Can you work these out from the model? Positions are in its coordinate system, mm. A direction names the side the tool comes from. Round coordinates to 2 decimals unless told otherwise and drop trailing zeros. Loops run counter-clockwise (first coordinate to the right, second up) from the corner with the lowest first, then second, coordinate; pieces in that order, holes last. Notation, with made-up numbers: (-24.75, -8) -> (-0.75, -8) arc R28 ccw to (-0.75, 23) -> close; hole circle Ø1 at (84, 24). An arc over 180 degrees is marked (long way). Write item = value, one per line.
from build123d import *

# Parameters (mm, degrees)
MAIN_EXTRUDE_DEPTH          = 2.2875
WALLS_START                 = 2.2875
WALLS_DEPTH                 = 13
CORNER_SUPPORT_DEPTH        = 2
FILLET4_R                   = 2
SKETCH4_W                   = 8.5
SKETCH4_H                   = 5.5
WIRE_HOLE_DEPTH             = 40.380356778
SKETCH25_W                  = 6
SKETCH25_H                  = 1.35
FEMALE_SNAP_DEPTH           = 10.125
SKETCH30_W                  = 15.7875
SKETCH30_H                  = 0.9
SKETCH30_W_2                = 17.7875
SKETCH30_H_2                = 1.5
MAGNET_EXTRUDE_1_DEPTH      = 7.625
MAGNET_EXTRUDE_1_DEPTH_BACK = 8.2
SKETCH29_R                  = 7.7
MAGNET_HOLE_DEPTH           = 2.1
SKETCH31_R                  = 5.5
MAGNET_THRU_HOLE_DEPTH      = 58.632218908
SKETCH40_W                  = 15.2875
SKETCH40_H                  = 12.55
CUT_EXTRUDE2_DEPTH          = 6
SKETCH41_W                  = 13
SKETCH41_H                  = 2
BOSS_EXTRUDE1_DEPTH         = 9.4


with BuildPart() as part:
    # Sketch1 → Main Extrude (new body)
    with BuildSketch(Plane(origin=(0, 0, 0), x_dir=(0, 0, -1), z_dir=(1, 0, 0))):
        Polygon((-30.5, -9.35), (-27.325, -9.35), (-27.325, -21.25), (28.5, -21.25), (28.5, 21.25), (-27.325, 21.25), (-27.325, 3.2), (-30.5, 3.2), align=None)
        with BuildLine():
            Line((20.7, -3.65), (-2.8, -3.65))
            ThreePointArc((-2.8, -3.65), (-4.6, -1.85), (-2.8, -0.05))
            Line((-2.8, -0.05), (20.7, -0.05))
            ThreePointArc((20.7, -0.05), (22.5, -1.85), (20.7, -3.65))
        make_face(mode=Mode.SUBTRACT)
    extrude(amount=MAIN_EXTRUDE_DEPTH)

    # Sketch1_3 → Walls (add)
    with BuildSketch(Plane(origin=(0, 0, 0), x_dir=(0, 0, -1), z_dir=(1, 0, 0)).offset(WALLS_START)):
        Polygon((-25.325, 19.25), (28.5, 19.25), (28.5, 21.25), (-27.325, 21.25), (-27.325, 3.2), (-30.5, 3.2), (-30.5, 1.3), (-25.325, 1.3), align=None)
        with BuildLine():
            Line((28.5, -5.425), (28, -5.425))
            ThreePointArc((28, -5.425), (26.939339828, -5.864339828), (26.5, -6.925))
            Line((26.5, -6.925), (26.5, -19.25))
            Line((26.5, -19.25), (-25.325, -19.25))
            Line((-25.325, -19.25), (-25.325, -8.1))
            Line((-25.325, -8.1), (-28.5, -8.1))
            Line((-28.5, -8.1), (-28.5, -4.45))
            Line((-28.5, -4.45), (-30.5, -4.45))
            Line((-30.5, -4.45), (-30.5, -9.35))
            Line((-30.5, -9.35), (-27.325, -9.35))
            Line((-27.325, -9.35), (-27.325, -21.25))
            Line((-27.325, -21.25), (28.5, -21.25))
            Line((28.5, -21.25), (28.5, -5.425))
        make_face()
    extrude(amount=WALLS_DEPTH)

    # Sketch22 → Corner Support (add)
    with BuildSketch(Plane(origin=(0, 0, -28.5), x_dir=(-1, 0, 0), z_dir=(0, 0, -1))):
        Polygon((-4.2875, 19.25), (-2.2875, 18.25), (-2.2875, 19.25), align=None)
    extrude(amount=-CORNER_SUPPORT_DEPTH)

    # Fillet4
    fillet4_edges = [part.edges().sort_by_distance(p)[0] for p in [
        (2.2875, -1.575, 30.5),
    ]]
    fillet(fillet4_edges, radius=FILLET4_R)

    # Sketch4 → Wire Hole (cut, through all)
    with BuildSketch(Plane(origin=(2.2875, 0, 0), x_dir=(0, 0, -1), z_dir=(1, 0, 0))):
        with Locations((22.25, -16.5)):
            Rectangle(SKETCH4_W, SKETCH4_H)
    extrude(amount=-WIRE_HOLE_DEPTH, mode=Mode.SUBTRACT)

    # Sketch25 → Female Snap (cut, symmetric)
    with BuildSketch(Plane(origin=(0, 0, -0.5875), x_dir=(-1, 0, 0), z_dir=(0, 0, -1))):
        with Locations((-11.0375, -19.925)):
            Rectangle(SKETCH25_W, SKETCH25_H)
        Polygon((-15.2875, -19.25), (-15.2875, -19.91463679), (-14.0375, -19.25), align=None)
        with Locations((-11.0375, 19.925)):
            Rectangle(SKETCH25_W, SKETCH25_H)
        Polygon((-15.2875, 19.91463679), (-15.2875, 19.25), (-14.0375, 19.25), align=None)
    extrude(amount=FEMALE_SNAP_DEPTH, both=True, mode=Mode.SUBTRACT)

    # Sketch30 → Magnet Extrude 1 (add, two sides)
    with BuildSketch(Plane(origin=(15.2875, 0, 0), x_dir=(0, 0, -1), z_dir=(1, 0, 0))) as magnet_extrude_1_sk:
        Polygon((-27.325, -18.35), (-27.325, -21.25), (-9.5375, -21.25), (-9.5375, -19.91463679), (-9.5375, -19.25), (-25.325, -19.25), (-25.325, -18.35), align=None)
        with Locations((-17.43125, -18.8)):
            Rectangle(SKETCH30_W, SKETCH30_H)
        with Locations((19.60625, -22)):
            Rectangle(SKETCH30_W_2, SKETCH30_H_2)
        Polygon((10.7125, -19.91463679), (10.7125, -21.25), (28.5, -21.25), (28.5, -18.35), (26.5, -18.35), (26.5, -19.25), (10.7125, -19.25), align=None)
        with Locations((-18.43125, -22)):
            Rectangle(SKETCH30_W_2, SKETCH30_H_2)
        with Locations((18.60625, -18.8)):
            Rectangle(SKETCH30_W, SKETCH30_H)
    extrude(amount=MAGNET_EXTRUDE_1_DEPTH)
    extrude(magnet_extrude_1_sk.sketch, amount=-MAGNET_EXTRUDE_1_DEPTH_BACK)

    # Sketch29 → Magnet Hole (cut)
    with BuildSketch(Plane(origin=(0, -21.95, 0), x_dir=(1, 0, 0), z_dir=(0, 1, 0))):
        with Locations((15.2875, -17.625)):
            Circle(SKETCH29_R)
        with BuildLine():
            ThreePointArc((22.9125, -18.697089082), (20.338980677, -23.436414885), (15.2875, -25.325))
            Line((15.2875, -25.325), (22.9125, -25.325))
            Line((22.9125, -25.325), (22.9125, -18.697089082))
        make_face()
        with BuildLine():
            Line((22.9125, -9.925), (15.2875, -9.925))
            ThreePointArc((15.2875, -9.925), (20.338980677, -11.813585115), (22.9125, -16.552910918))
            Line((22.9125, -16.552910918), (22.9125, -9.925))
        make_face()
        with Locations((15.2875, 19.4)):
            Circle(SKETCH29_R)
        with BuildLine():
            ThreePointArc((22.9125, 18.327910918), (20.338980677, 13.588585115), (15.2875, 11.7))
            Line((15.2875, 11.7), (22.9125, 11.7))
            Line((22.9125, 11.7), (22.9125, 18.327910918))
        make_face()
        with BuildLine():
            Line((22.9125, 27.1), (15.2875, 27.1))
            ThreePointArc((15.2875, 27.1), (20.338980677, 25.211414885), (22.9125, 20.472089082))
            Line((22.9125, 20.472089082), (22.9125, 27.1))
        make_face()
        with BuildLine():
            ThreePointArc((22.9875, -17.625), (22.968727116, -17.087645368), (22.9125, -16.552910918))
            Line((22.9125, -16.552910918), (22.9125, -18.697089082))
            ThreePointArc((22.9125, -18.697089082), (22.968727116, -18.162354632), (22.9875, -17.625))
        make_face()
        with BuildLine():
            Line((22.9125, 20.472089082), (22.9125, 18.327910918))
            ThreePointArc((22.9125, 18.327910918), (22.968727116, 18.862645368), (22.9875, 19.4))
            ThreePointArc((22.9875, 19.4), (22.968727116, 19.937354632), (22.9125, 20.472089082))
        make_face()
    extrude(amount=MAGNET_HOLE_DEPTH, mode=Mode.SUBTRACT)

    # Sketch31 → Magnet Thru Hole (cut, through all)
    with BuildSketch(Plane.XZ.offset(21.95)):
        with Locations((15.2875, 17.625)):
            Circle(SKETCH31_R)
        with BuildLine():
            Line((22.9125, 23.125), (15.2875, 23.125))
            ThreePointArc((15.2875, 23.125), (19.176587297, 21.514087297), (20.7875, 17.625))
            ThreePointArc((20.7875, 17.625), (19.176587297, 13.735912703), (15.2875, 12.125))
            Line((15.2875, 12.125), (22.9125, 12.125))
            Line((22.9125, 12.125), (22.9125, 23.125))
        make_face()
        with Locations((15.2875, -19.4)):
            Circle(SKETCH31_R)
        with BuildLine():
            Line((22.9125, -13.9), (15.2875, -13.9))
            ThreePointArc((15.2875, -13.9), (19.176587297, -15.510912703), (20.7875, -19.4))
            ThreePointArc((20.7875, -19.4), (19.176587297, -23.289087297), (15.2875, -24.9))
            Line((15.2875, -24.9), (22.9125, -24.9))
            Line((22.9125, -24.9), (22.9125, -13.9))
        make_face()
    extrude(amount=MAGNET_THRU_HOLE_DEPTH, mode=Mode.SUBTRACT)

    # Sketch40 → Cut-Extrude2 (cut)
    with BuildSketch(Plane.XY.offset(27.325)):
        with Locations((7.64375, -3.075)):
            Rectangle(SKETCH40_W, SKETCH40_H)
    extrude(amount=CUT_EXTRUDE2_DEPTH, mode=Mode.SUBTRACT)

    # Sketch41 → Boss-Extrude1 (add)
    with BuildSketch(Plane.XZ.offset(-1.3)):
        with Locations((8.7875, 26.325)):
            Rectangle(SKETCH41_W, SKETCH41_H)
    extrude(amount=BOSS_EXTRUDE1_DEPTH)


solid = part.part
1. I'm going to push flat-ended pins straight in: pin 1 (0.7 mm diameter, centred on y = -19, z = 14, fed in from -X); pin 2 (20 mm diameter, centred on y = 3.5, z = -9.5, fed in from +X); pin 3 (3 mm diameter, centred on x = 3.5, z = 12.5, fed in from -Y); pin 4 (0.7 mm diameter, centred on y = 20, z = -4, fed in from +X). Where does each tip first touch, or does it pass through?
Entries:
pin_1 = 0
pin_2 = 2.29
pin_3 = -21.25
pin_4 = 15.29
2. Suppose I cut it at B-B, the plane z = -19.4. List the corners of the cut face in (x, y) for me.
Entries:
outline = (0, -21.25) -> (7.09, -21.25) -> (7.09, -22.75) -> (9.79, -22.75) -> (9.79, -21.95) -> (7.59, -21.95) -> (7.59, -19.85) -> (22.91, -19.85) -> (22.91, -18.35) -> (7.09, -18.35) -> (7.09, -19.25) -> (0, -19.25) -> close; (0, -13.75) -> (2.29, -13.75) -> (2.29, -3.65) -> (0, -3.65) -> close; (0, -0.05) -> (2.29, -0.05) -> (2.29, 19.25) -> (15.29, 19.25) -> (15.29, 21.25) -> (0, 21.25) -> close
3. Suppose I cut it at C-C, the plane y = -1.85. List the corners of the cut face in (x, z) for me (1 decimal), and give its area (3 significant figures).
Entries:
outline = (0, -28.5) -> (2.3, -28.5) -> (2.3, -22.5) -> (0, -22.5) -> close; (0, 4.6) -> (2.3, 4.6) -> (2.3, 25.3) -> (15.3, 25.3) -> (15.3, 27.3) -> (0, 27.3) -> close
area = 91.7 mm²
4. We'd pull the mould along X, two halves only. Please class faces 1 (the flat face through (15.288, -12, -27)), 2 (the flat face through (15, -19.85, -20)), 3 (the flat face through (8.038, 20, -1)): released by +X, released by -X, zero draft, split by the parting line, or undercut.
Entries:
face_1 = released by +X
face_2 = zero draft
face_3 = undercut
5. I need wall thicknesses on line 1 (Y direction, x = 13, z = -23); line 2 (Y direction, x = 3, z = 9.5); line 3 (Y direction, x = 8.5, z = 17). Which ranges of each line are inside material? Lowest first, please. Write a range as [from, to].
Entries:
line_1 = [-19.85, -18.35], [19.25, 21.25]
line_2 = [-21.25, -19.25], [19.25, 21.25]
line_3 = [-22.75, -21.95], [-19.85, -18.35], [19.25, 21.25]
6. Suppose I cut it at D-D, the plane z = -8. List the corners of the cut face in (x, y) for me.
Entries:
outline = (0, -21.25) -> (15.29, -21.25) -> (15.29, -19.91) -> (14.04, -19.25) -> (14.04, -20.6) -> (8.04, -20.6) -> (8.04, -19.25) -> (2.29, -19.25) -> (2.29, -3.65) -> (0, -3.65) -> close; (0, -0.05) -> (2.29, -0.05) -> (2.29, 19.25) -> (8.04, 19.25) -> (8.04, 20.6) -> (14.04, 20.6) -> (14.04, 19.25) -> (15.29, 19.91) -> (15.29, 21.25) -> (0, 21.25) -> close
7. For faces 4 (the flat face through (1, -17, -18)), 5 (the flat face through (19, -21, -11.7)), 6 (the flat face through (14.038, -20, 0)), 7 (the cylindrical face through (1.1, -1.8, -22.5)), 8 (the flat face through (7.088, -22, -19)), which set-ups out of +Z, -Z, +X, -X, +Y, -Y let a thin tool reach every point of the face, with its end or its side?
Entries:
face_4 = -X
face_5 = +X
face_6 = none
face_7 = +X, -X
face_8 = +Z, -Z, -X, -Y
